The model under review builds one solid part; all positions refer to its coordinate system, in mm. A direction names the side the tool comes from. Coordinates: 2 decimals unless noted, no trailing zeros. Order: outer loops, then holes, each group sorted by start corner. A loop starts at its lowest first (then second) coordinate and runs counter-clockwise, first axis right, second up. Notation, with made-up numbers: M 47,-39.5 L 85,-39.5 A23 ccw 85,-4.5 Z; hole C 40,31.5 d3. An arc over 180 degrees is marked long. One line per item, written item: value.
```python
from build123d import *

# Parameters (mm, degrees)
BOSS_EXTRUDE1_DEPTH = 3
SKETCH3_R           = 7.5
CUT_EXTRUDE1_DEPTH  = 10
SKETCH4_W           = 3
SKETCH4_H           = 20
BOSS_EXTRUDE2_DEPTH = 3


with BuildPart() as part:
    # Sketch1 → Boss-Extrude1 (new body)
    with BuildSketch(Plane.XY):
        Polygon((-10, 52), (-10, 55), (10, 55), (10, 52), (30, 52), (30, -52), (10, -52), (10, -55), (-10, -55), (-10, -52), (-27, -52), (-27, 52), align=None)
    extrude(amount=BOSS_EXTRUDE1_DEPTH)

    # Sketch3 → Cut-Extrude1 (cut)
    with BuildSketch(Plane.XY.offset(3)):
        with Locations((-14.432858662, 0)):
            Circle(SKETCH3_R)
    extrude(amount=-CUT_EXTRUDE1_DEPTH, mode=Mode.SUBTRACT)

    # Sketch4 → Boss-Extrude2 (add)
    with BuildSketch(Plane.ZY.offset(27)):
        with Locations((1.5, 0)):
            Rectangle(SKETCH4_W, SKETCH4_H)
    extrude(amount=BOSS_EXTRUDE2_DEPTH)


solid = part.part
```
(1) For L1, parallel to X at y = -0.5, z = 2.15; L2, parallel to X at y = 29, z = 0.25; L3, parallel to Y at x = 16, z = 2.4, list the stretches that pass through material, from the lowest coordinate up.
Geometry results:
L1: x = -30 to -21.92, -6.95 to 30
L2: x = -27 to 30
L3: y = -52 to 52
(2) Tool access review of faces 1 (the flat face through (-10, -54, 1)), 2 (the flat face through (10, 54, 1)), 3 (the flat face through (-10, 53, 1)): name each direction out of +Z, -Z, +X, -X, +Y, -Y from which nothing blocks a thin tool from reaching the whole face with its end or side.
Geometry results:
face 1: +Z, -Z, -X, -Y
face 2: +Z, -Z, +X, +Y
face 3: +Z, -Z, -X, +Y
(3) We need section C-C, the plane y = 39.5. State the section outline as (x, z) points, plus the area to 3 significant figures.
Geometry results:
outline: M -27,0 L 30,0 L 30,3 L -27,3 Z
area: 171 mm2
(4) We need section B-B, the plane z = 1.1. State the section outline as (x, y) points.
Geometry results:
outline: M -30,-10 L -27,-10 L -27,-52 L -10,-52 L -10,-55 L 10,-55 L 10,-52 L 30,-52 L 30,52 L 10,52 L 10,55 L -10,55 L -10,52 L -27,52 L -27,10 L -30,10 Z; hole C -14.43,0 d15
(5) Insertion check: pin 1 Ø1.5 at (y, z) = (-53, 1.5) entering from -X; pin 2 Ø0.9 at (x, z) = (19, 2) entering from -Y; pin 3 Ø1.5 at (y, z) = (54, 1.5) entering from +X. Each pin has a flat end and moves straight along its axis. Give the tip position at first contact, or say it passes through.
Geometry results:
pin 1: stops at x = -10
pin 2: stops at y = -52
pin 3: stops at x = 10
(6) We need section A-A, the plane y = 5. State the section outline as (x, z) points.
Geometry results:
outline: M -30,0 L -20.02,0 L -20.02,3 L -30,3 Z; M -8.84,0 L 30,0 L 30,3 L -8.84,3 Z
(7) We need section D-D, the plane y = -6. State the section outline as (x, z) points, plus the area to 3 significant figures.
Geometry results:
outline: M -30,0 L -18.93,0 L -18.93,3 L -30,3 Z; M -9.93,0 L 30,0 L 30,3 L -9.93,3 Z
area: 153 mm2
